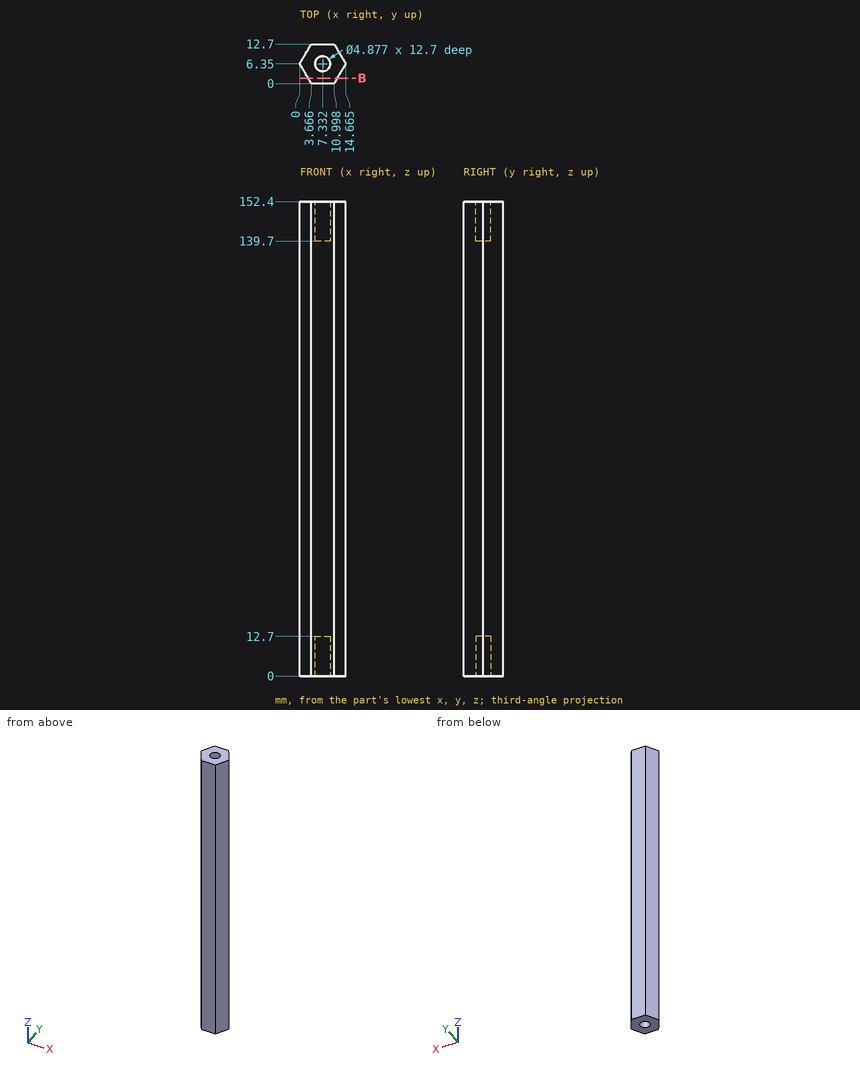
Design review of the part shown in the three views and the two pictorial views. Dimensions are in mm from the part's minimum x, y and z. Coordinates: 2 decimals unless noted, no trailing zeros. Write each loop counter-clockwise with the first axis right and the second up, starting at its lowest first coordinate (ties: lowest second). Pieces come first, ordered by that corner, then holes.
1) We need section B-B on y = 1.75. State the section outline as (x, z) points (1 decimal), then the cut area to 3 significant figures.
2) Clearance check with flat-ended pins moving along their axes: pin 1 Ø3 at (x, y) = (7.33, 6.35) entering from -Z; pin 2 Ø6 at (y, z) = (7, 107) entering from -X; pin 3 Ø1.5 at (x, z) = (2.5, 129) entering from +Y. State where each tip first meets the part, or that it passes through.
3) To check wall thickness, follow probe 1 along Y at (x, z) = (12.5, 33) (1 decimal); probe 2 along X at (y, z) = (5.75, 28.5) (1 decimal); probe 3 along Y at (x, z) = (0.5, 95) (1 decimal). State the ranges of each line that lie inside material, in increasing order.
Answer list:
1. outline: (2.7, 0) - (12, 0) - (12, 152.4) - (2.7, 152.4) - close
1. area: 1,430 mm2
2. pin 1: stops at z = 12.7
2. pin 2: stops at x = 0
2. pin 3: stops at y = 11.98
3. probe 1: y = 2.6 to 10.1
3. probe 2: x = 0.3 to 14.3
3. probe 3: y = 5.5 to 7.2
